Work out the finished part from the listing and answer in its coordinate system (mm). Face numbers are marked on the shaded views. A direction names the side the tool comes from. Coordinates: 2 decimals unless noted, no trailing zeros. Use a Markdown table: item, result.
from build123d import *

# Parameters (mm, degrees)
F0_W      = 48.8188
F0_H      = 31.496
F1_DEPTH  = 3.20802
F2_R      = 2.413
F3_DEPTH  = 1.778
F4_DEPTH  = 1.778
F5_DEPTH  = 1.778
F6_DEPTH  = 1.778
F7_DEPTH  = 1.778
F8_DEPTH  = 1.778
F9_T      = -1.5748
F10_R     = 3.2131
F10_R_2   = 2.6224244876
F10_R_3   = 2.5317158825
F10_R_4   = 2.613200879
F11_DEPTH = 1.4563


with BuildPart() as f1:
    # F0 (on Top) → F1 (new body)
    with BuildSketch(Plane.XY):
        with Locations((24.4094, 15.748)):
            Rectangle(F0_W, F0_H)
    extrude(amount=F1_DEPTH)

    # F2 (on face) → F3 (join)
    with BuildSketch(Plane.XY.offset(3.20802)):
        with Locations((3.9209306593, 27.559)):
            Circle(F2_R)
    extrude(amount=F3_DEPTH)

    # F2 (on face) → F4 (join)
    with BuildSketch(Plane.XY.offset(3.20802)):
        with Locations((11.7949306593, 27.559)):
            Circle(F2_R)
    extrude(amount=F4_DEPTH)

    # F2 (on face) → F5 (join)
    with BuildSketch(Plane.XY.offset(3.20802)):
        with Locations((19.6689306593, 27.559)):
            Circle(F2_R)
    extrude(amount=F5_DEPTH)

    # F2 (on face) → F6 (join)
    with BuildSketch(Plane.XY.offset(3.20802)):
        with Locations((27.5429306593, 27.559)):
            Circle(F2_R)
    extrude(amount=F6_DEPTH)

    # F2 (on face) → F7 (join)
    with BuildSketch(Plane.XY.offset(3.20802)):
        with Locations((35.4169306593, 27.559)):
            Circle(F2_R)
    extrude(amount=F7_DEPTH)

    # F2 (on face) → F8 (join)
    with BuildSketch(Plane.XY.offset(3.20802)):
        with Locations((43.2909306593, 27.559)):
            Circle(F2_R)
        with Locations((3.9209306593, 19.685)):
            Circle(F2_R)
        with Locations((11.7949306593, 19.685)):
            Circle(F2_R)
        with Locations((19.6689306593, 19.685)):
            Circle(F2_R)
        with Locations((27.5429306593, 19.685)):
            Circle(F2_R)
        with Locations((35.4169306593, 19.685)):
            Circle(F2_R)
        with Locations((43.2909306593, 19.685)):
            Circle(F2_R)
        with Locations((43.2909306593, 11.811)):
            Circle(F2_R)
        with Locations((35.4169306593, 11.811)):
            Circle(F2_R)
        with Locations((27.5429306593, 11.811)):
            Circle(F2_R)
        with Locations((19.6689306593, 11.811)):
            Circle(F2_R)
        with Locations((11.7949306593, 11.811)):
            Circle(F2_R)
        with Locations((3.9209306593, 11.811)):
            Circle(F2_R)
        with Locations((3.9209306593, 3.937)):
            Circle(F2_R)
        with Locations((11.7949306593, 3.937)):
            Circle(F2_R)
        with Locations((19.6689306593, 3.937)):
            Circle(F2_R)
        with Locations((27.5429306593, 3.937)):
            Circle(F2_R)
        with Locations((35.4169306593, 3.937)):
            Circle(F2_R)
        with Locations((43.2909306593, 3.937)):
            Circle(F2_R)
    extrude(amount=F8_DEPTH)

    # F9
    f9_openings = [f1.faces().sort_by_distance(p)[0] for p in [
        (24.4094, 15.748, 0),
    ]]
    offset(amount=F9_T, openings=f9_openings, kind=Kind.INTERSECTION)

    # F10 (on face) → F11 (join)
    with BuildSketch(Plane(origin=(0, 0, 1.63322), x_dir=(1, 0, 0), z_dir=(0, 0, -1))):
        with Locations((15.7772629731, -7.8114119043)):
            Circle(F10_R)
        with Locations((15.7772629731, -7.8114119043)):
            Circle(F10_R_2, mode=Mode.SUBTRACT)
        with Locations((7.9032629731, -7.8114119043)):
            Circle(F10_R)
        with Locations((7.9032629731, -7.8114119043)):
            Circle(F10_R_2, mode=Mode.SUBTRACT)
        with Locations((23.6512629731, -7.8114119043)):
            Circle(F10_R)
        with Locations((23.6512629731, -7.8114119043)):
            Circle(F10_R_2, mode=Mode.SUBTRACT)
        with Locations((31.5252629731, -7.8114119043)):
            Circle(F10_R)
        with Locations((31.5252629731, -7.8114119043)):
            Circle(F10_R_2, mode=Mode.SUBTRACT)
        with Locations((39.3992629731, -7.8114119043)):
            Circle(F10_R)
        with Locations((39.3992629731, -7.8114119043)):
            Circle(F10_R_2, mode=Mode.SUBTRACT)
        with Locations((39.3992629731, -15.8124119043)):
            Circle(F10_R)
        with Locations((39.3992629731, -15.8124119043)):
            Circle(F10_R_3, mode=Mode.SUBTRACT)
        with Locations((31.5252629731, -15.8124119043)):
            Circle(F10_R)
        with Locations((31.5252629731, -15.8124119043)):
            Circle(F10_R_3, mode=Mode.SUBTRACT)
        with Locations((23.6512629731, -15.8124119043)):
            Circle(F10_R)
        with Locations((23.6512629731, -15.8124119043)):
            Circle(F10_R_3, mode=Mode.SUBTRACT)
        with Locations((15.7772629731, -15.8124119043)):
            Circle(F10_R)
        with Locations((15.7772629731, -15.8124119043)):
            Circle(F10_R_3, mode=Mode.SUBTRACT)
        with Locations((7.9032629731, -15.8124119043)):
            Circle(F10_R)
        with Locations((7.9032629731, -15.8124119043)):
            Circle(F10_R_3, mode=Mode.SUBTRACT)
        with Locations((7.9032629731, -23.8134119043)):
            Circle(F10_R)
        with Locations((7.9032629731, -23.8134119043)):
            Circle(F10_R_4, mode=Mode.SUBTRACT)
        with Locations((15.7772629731, -23.8134119043)):
            Circle(F10_R)
        with Locations((15.7772629731, -23.8134119043)):
            Circle(F10_R_4, mode=Mode.SUBTRACT)
        with Locations((23.6512629731, -23.8134119043)):
            Circle(F10_R)
        with Locations((23.6512629731, -23.8134119043)):
            Circle(F10_R_4, mode=Mode.SUBTRACT)
        with Locations((31.5252629731, -23.8134119043)):
            Circle(F10_R)
        with Locations((31.5252629731, -23.8134119043)):
            Circle(F10_R_4, mode=Mode.SUBTRACT)
        with Locations((39.3992629731, -23.8134119043)):
            Circle(F10_R)
        with Locations((39.3992629731, -23.8134119043)):
            Circle(F10_R_4, mode=Mode.SUBTRACT)
    extrude(amount=F11_DEPTH)


solid = f1.part
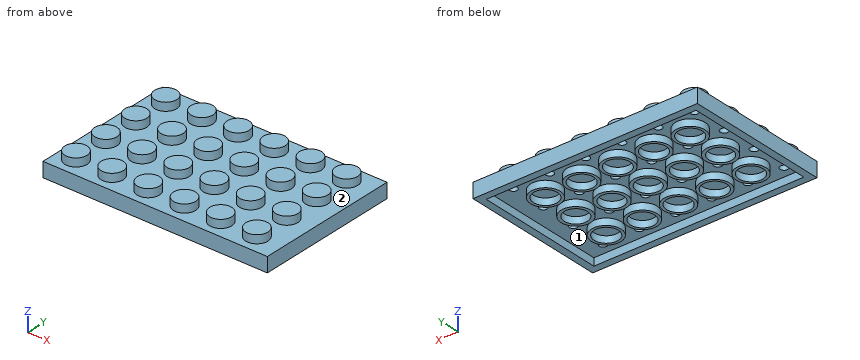
(1) A cutting plane is placed at A-A (z = 4.1). Give the number of separate pieces and of enclosed holes in the cut face, then the cut area to 3 significant figures.
Conclusion:
| item | result |
|---|---|
| separate pieces | 24 |
| enclosed holes | 0 |
| area | 439 mm2 |
(2) Given P1, Ø5.5, axis at x = 32, y = 15.5, coming from the -Z side; P2, Ø0.8, axis at x = 28, y = 3.5, coming from the -Z side; P3, Ø1, axis at x = 35.42, y = 3.94, coming from the -Z side, each flat-ended and moving along its own axis, determine where each tip first touches the part or whether it passes through.
Conclusion:
| item | result |
|---|---|
| P1 | z = 0.18 |
| P2 | z = 1.63 |
| P3 | z = 3.41 |
(3) Straight lines are drawn through the part: L1, parallel to X at y = 19.5, z = 4.75; L2, parallel to Y at x = 19.5, z = 4.7; L3, parallel to Y at x = 35, z = 2.2. For each, find the intervals that lie inside material, in ascending order.
Conclusion:
| item | result |
|---|---|
| L1 | 1.52 to 6.33, 9.39 to 14.2, 17.26 to 22.07, 25.14 to 29.95, 33.01 to 37.82, 40.89 to 45.7 |
| L2 | 1.53 to 6.34, 9.4 to 14.22, 17.28 to 22.09, 25.15 to 29.97 |
| L3 | 0 to 3.21, 4.66 to 11.08, 12.54 to 18.96, 20.41 to 26.83, 28.29 to 31.5 |
(4) Which of the six approach directions +Z, -Z, +X, -X, +Y, -Y give full straight-line access (tool end or side, diameter ignored) to the marked faces 1 and 2?
Conclusion:
| item | result |
|---|---|
| face 1 | -Z |
| face 2 | +Z |
